from build123d import *

# Parameters (mm, degrees)
SKETCH1_W           = 20
SKETCH1_H           = 20
BOSS_EXTRUDE1_DEPTH = 2
SKETCH4_R           = 3
BOSS_EXTRUDE2_DEPTH = 1


with BuildPart() as part:
    # Sketch1 → Boss-Extrude1 (new body)
    with BuildSketch(Plane(origin=(0, 0, 0), x_dir=(1, 0, 0), z_dir=(0, 1, 0))):
        Rectangle(SKETCH1_W, SKETCH1_H)
    extrude(amount=BOSS_EXTRUDE1_DEPTH)

    # Sketch4 → Boss-Extrude2 (add)
    with BuildSketch(Plane.XY.offset(5)):
        with BuildLine():
            Line((-7.5, 17), (-7.5, 2))
            Line((-7.5, 2), (7.5, 2))
            Line((7.5, 2), (7.5, 17))
            ThreePointArc((7.5, 17), (0, 24.5), (-7.5, 17))
        make_face()
        with Locations((0, 17)):
            Circle(SKETCH4_R, mode=Mode.SUBTRACT)
    boss_extrude2 = extrude(amount=BOSS_EXTRUDE2_DEPTH)

    # Mirror1: Boss-Extrude2 across plane
    add(boss_extrude2.mirror(Plane.XY))


solid = part.part
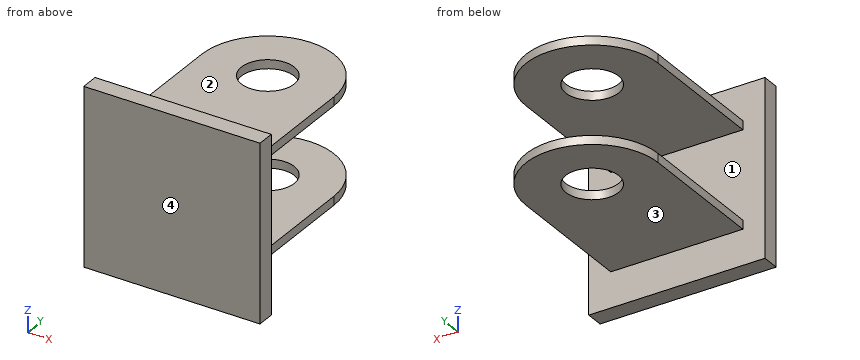
The model under review builds one solid part; all positions refer to its coordinate system, in mm. Face numbers are marked on the shaded views. Round coordinates to 2 decimals unless told otherwise and drop trailing zeros. Loops run counter-clockwise (first coordinate to the right, second up) from the corner with the lowest first, then second, coordinate; pieces in that order, holes last. Notation, with made-up numbers: M 71,9.25 L 76,9.25 A28 ccw 76,36.25 Z; hole C 28,45.5 d1. An arc over 180 degrees is marked long. Answer as CSV lines item,"result". Start each with the question number.
Item 1: Consider section C-C (x = -5). Write out the cut boundary in (y, z).
Item 2: Consider section B-B (y = 17.75). Write out the cut boundary in (x, z).
Item 3: Insertion check: P1, Ø5, axis at x = 0, y = 17, coming from the +Z side; P2, Ø6, axis at y = 15, z = -3.5, coming from the -X side; P3, Ø0.5, axis at y = 6, z = 5.5, coming from the +X side; P4, Ø7, axis at x = 0, y = 17, coming from the +Z side. Each pin has a flat end and moves straight along its axis. Give the tip position at first contact, or say it passes through.
Item 4: Mouldability with a two-part tool opening along Z and no side actions: class the marked faces 1, 2, 3 and 4 as released by +Z, released by -Z, zero draft, split by the parting line, or undercut.
Item 5: Consider section D-D (z = -3.5). Write out the cut boundary in (x, y), then the cut area to 3 significant figures.
Item 6: Wall thickness on line 1 (Z direction, x = 3.25, y = 2.25); line 2 (Y direction, x = 0, z = -5.5); line 3 (Y direction, x = -0.25, z = 7.75): over which ranges is each line inside the solid? List them lowest first. Write a range as [from, to].
Item 7: Consider section A-A (x = 0). Write out the cut boundary in (y, z).
Answer:
1,outline,"M 0,-10 L 2,-10 L 2,-6 L 22.59,-6 L 22.59,-5 L 2,-5 L 2,5 L 22.59,5 L 22.59,6 L 2,6 L 2,10 L 0,10 Z"
2,outline,"M -7.46,-6 L -2.9,-6 L -2.9,-5 L -7.46,-5 Z; M -7.46,5 L -2.9,5 L -2.9,6 L -7.46,6 Z; M 2.9,-6 L 7.46,-6 L 7.46,-5 L 2.9,-5 Z; M 2.9,5 L 7.46,5 L 7.46,6 L 2.9,6 Z"
3,P1,"passes through"
3,P2,"stops at x = -7.5"
3,P3,"stops at x = 7.5"
3,P4,"stops at z = 6"
4,face 1,"undercut"
4,face 2,"released by +Z"
4,face 3,"released by -Z"
4,face 4,"zero draft"
5,outline,"M -10,0 L 10,0 L 10,2 L -10,2 Z"
5,area,"40.0 mm^2"
6,line 1,"z = [-6, -5], [5, 6]"
6,line 2,"y = [0, 14], [20, 24.5]"
6,line 3,"y = [0, 2]"
7,outline,"M 0,-10 L 2,-10 L 2,-6 L 14,-6 L 14,-5 L 2,-5 L 2,5 L 14,5 L 14,6 L 2,6 L 2,10 L 0,10 Z; M 20,-6 L 24.5,-6 L 24.5,-5 L 20,-5 Z; M 20,5 L 24.5,5 L 24.5,6 L 20,6 Z"
